from build123d import *

# Parameters (mm, degrees)
EXTRUDE003_DEPTH                     = 10
SKETCH009_R                          = 3.1
EXTRUDE002_DEPTH                     = 10
EXTRUDE001_DEPTH                     = 2.65
EXTRUDE001_ONTO_SKETCH005_ROLL_ANGLE = 90
EXTRUDE_DEPTH                        = 30
EXTRUDE_ONTO_SKETCH_ROLL_ANGLE       = 90
POCKET_DEPTH                         = 20.000966
SKETCH002_W                          = 9.15
SKETCH002_H                          = 3.1
POCKET001_DEPTH                      = 7
POCKET002_DEPTH                      = 3.739432
SKETCH004_R                          = 1.55
POCKET003_DEPTH                      = 7
SKETCH006_W                          = 6
SKETCH006_H                          = 4
POCKET004_DEPTH                      = 9.5
SKETCH007_R                          = 4.15
POCKET005_DEPTH                      = 14.611568
FILLET_R                             = 2.5
FILLET001_R                          = 1
FILLET002_R                          = 2
FILLET003_R                          = 1
CHAMFER_1_SIZE2                      = 16
CHAMFER_1_SIZE                       = 6
CHAMFER_2_SIZE2                      = 16
CHAMFER_2_SIZE                       = 6
CHAMFER001_SIZE                      = 5
SKETCH008_R                          = 1.55
POCKET006_DEPTH                      = 5.826
POCKET006_DEPTH_BACK                 = 6.476
FILLET004_R                          = 5


with BuildPart() as extrude003:
    # Sketch010 → Extrude003 (new body)
    with BuildSketch(Plane(origin=(0.325, 0, 0), x_dir=(0, -1, 0), z_dir=(-1, 0, 0))):
        Polygon((-21.103517, 11.668627), (-23.788196, 10.118627), (-23.788196, 7.018627), (-21.103517, 5.468627), (-18.418839, 7.018627), (-18.418839, 10.118627), align=None)
    extrude(amount=-EXTRUDE003_DEPTH)


with BuildPart() as extrude003_1:
    # Extrude003 placement: moved
    add(extrude003.part.moved(Location((2, 0, 0))))


with BuildPart() as extrude002:
    # Sketch009 → Extrude002 (new body)
    with BuildSketch(Plane.YZ.offset(-0.325)):
        with Locations((21.103517, 8.568627)):
            Circle(SKETCH009_R)
    extrude(amount=-EXTRUDE002_DEPTH)


with BuildPart() as extrude002_1:
    # Extrude002 placement: moved
    add(extrude002.part.moved(Location((-2, 0, 0))))


with BuildPart() as extrude001:
    # Sketch005 as drawn → Extrude001 (new)
    with BuildSketch(Plane.XY):
        Polygon((-2.75, -6.999966), (2.75, -6.999966), (2.75, -1.912252), (0, -0.324539), (-2.75, -1.912252), align=None)
    extrude(amount=-EXTRUDE001_DEPTH)


with BuildPart() as extrude001_1:
    # Extrude001 onto Sketch005 roll: moved
    add(extrude001.part.rotate(Axis((0, 0, 0), (1, 0, 0)), EXTRUDE001_ONTO_SKETCH005_ROLL_ANGLE))


with BuildPart() as extrude001_2:
    # Extrude001 onto Sketch005 placement: moved
    add(extrude001_1.part.moved(Location((0, 3.738432, 0))))


with BuildPart() as extrude001_3:
    # Extrude001 placement: moved
    add(extrude001_2.part.moved(Location((0, 3, 0))))


with BuildPart() as cut002:
    # Sketch as drawn → Extrude (new)
    with BuildSketch(Plane.XY):
        with BuildLine():
            ThreePointArc((-5.994013, 1.376339), (-6.110877, 0.692592), (-6.15, 3.4e-05))
            Line((-6.15, 3.4e-05), (-6.15, -6.999966))
            Line((-6.15, -6.999966), (6.15, -6.999966))
            Line((6.15, -6.999966), (6.15, 0))
            ThreePointArc((6.15, 0), (6.110879, 0.692575), (5.994013, 1.376339))
            Line((5.994013, 1.376339), (3.325, 13))
            Line((3.325, 13), (0.325, 13))
            Line((0.325, 13), (0.325, 0.945714))
            ThreePointArc((-0.325, 0.945714), (0, -1), (0.325, 0.945714))
            Line((-0.325, 13), (-0.325, 0.945714))
            Line((-3.325, 13), (-0.325, 13))
            Line((-5.994013, 1.376339), (-3.325, 13))
        make_face()
    extrude(amount=-EXTRUDE_DEPTH)


with BuildPart() as cut002_1:
    # Extrude onto Sketch roll: moved
    add(cut002.part.rotate(Axis((0, 0, 0), (1, 0, 0)), EXTRUDE_ONTO_SKETCH_ROLL_ANGLE))


with BuildPart() as cut002_2:
    # Extrude onto Sketch placement: moved
    add(cut002_1.part)

    # Sketch001 → Pocket (cut, through all)
    with BuildSketch(Plane(origin=(0, 0, -6.999966), x_dir=(1, 0, 0), z_dir=(0, 0, -1))):
        with BuildLine():
            Line((-6.15, 0), (6.15, 0))
            ThreePointArc((-6.15, 0), (0, -1.390023), (6.15, 0))
        make_face()
    extrude(amount=-POCKET_DEPTH, mode=Mode.SUBTRACT)

    # Sketch002 → Pocket001 (cut)
    with BuildSketch(Plane(origin=(0, 0, -6.999966), x_dir=(1, 0, 0), z_dir=(0, 0, -1))):
        with Locations((0, -2.188432)):
            Rectangle(SKETCH002_W, SKETCH002_H)
    extrude(amount=-POCKET001_DEPTH, mode=Mode.SUBTRACT)

    # Sketch003 → Pocket002 (cut, through all)
    with BuildSketch(Plane.XZ.offset(-3.738432)):
        Polygon((4.575, 3.4e-05), (-4.575, 3.4e-05), (0, 2.641412), align=None)
    extrude(amount=POCKET002_DEPTH, mode=Mode.SUBTRACT)

    # Sketch004 → Pocket003 (cut)
    with BuildSketch(Plane.XZ.offset(-3.738432)):
        with Locations((0, -3.499966)):
            Circle(SKETCH004_R)
    extrude(amount=-POCKET003_DEPTH, mode=Mode.SUBTRACT)

    # Cut: cut Extrude001
    add(extrude001_3.part, mode=Mode.SUBTRACT)

    # Sketch006 → Pocket004 (cut)
    with BuildSketch(Plane(origin=(0, 0, -6.999966), x_dir=(1, 0, 0), z_dir=(0, 0, -1))):
        with Locations((0, -13.388432)):
            Rectangle(SKETCH006_W, SKETCH006_H)
    extrude(amount=-POCKET004_DEPTH, mode=Mode.SUBTRACT)

    # Sketch007 → Pocket005 (cut)
    with BuildSketch(Plane(origin=(0, 30, 0), x_dir=(-1, 0, 0), z_dir=(0, 1, 0))):
        Circle(SKETCH007_R)
    extrude(amount=-POCKET005_DEPTH, mode=Mode.SUBTRACT)

    # Fillet
    fillet_edges = [cut002_2.edges().sort_by_distance(p)[0] for p in [
        (3, 13.388432, 2.500034),
        (-3, 13.388432, 2.500034),
    ]]
    fillet(fillet_edges, radius=FILLET_R)

    # Fillet001
    fillet001_edges = [cut002_2.edges().sort_by_distance(p)[0] for p in [
        (3, 11.388432, -3.499966),
        (2.267767, 11.388432, 1.767801),
        (0.4125, 11.388432, 2.500034),
        (-3, 11.388432, -3.499966),
        (-2.267767, 11.388432, 1.767801),
        (-0.4125, 11.388432, 2.500034),
    ]]
    fillet(fillet001_edges, radius=FILLET001_R)

    # Fillet002
    fillet002_edges = [cut002_2.edges().sort_by_distance(p)[0] for p in [
        (0, 15.388432, -4.15),
    ]]
    fillet(fillet002_edges, radius=FILLET002_R)

    # Fillet003
    fillet003_edges = [cut002_2.edges().sort_by_distance(p)[0] for p in [
        (3, 13.888432, -6.999966),
        (0, 15.388432, -6.999966),
        (2.707107, 11.681325, -6.999966),
        (0, 11.388432, -6.999966),
        (-3, 13.888432, -6.999966),
        (-2.707107, 11.681325, -6.999966),
    ]]
    fillet(fillet003_edges, radius=FILLET003_R)

    # Chamfer 1
    chamfer_1_edges = [cut002_2.edges().sort_by_distance(p)[0] for p in [
        (1.835295, 1.271761, 13),
    ]]
    chamfer_1_side = cut002_2.faces().sort_by_distance((3.310874, 1.001462, 3.000017))[0]
    chamfer(chamfer_1_edges, length=CHAMFER_1_SIZE, length2=CHAMFER_1_SIZE2, reference=chamfer_1_side)

    # Chamfer 2
    chamfer_2_edges = [cut002_2.edges().sort_by_distance(p)[0] for p in [
        (-1.835295, 1.271761, 13),
    ]]
    chamfer_2_side = cut002_2.faces().sort_by_distance((-3.310874, 1.001462, 3.000017))[0]
    chamfer(chamfer_2_edges, length=CHAMFER_2_SIZE, length2=CHAMFER_2_SIZE2, reference=chamfer_2_side)

    # Chamfer001
    chamfer001_edges = [cut002_2.edges().sort_by_distance(p)[0] for p in [
        (1.825, 30, 13),
        (-1.825, 30, 13),
    ]]
    chamfer(chamfer001_edges, length=CHAMFER001_SIZE)

    # Sketch008 → Pocket006 (cut, two sides)
    with BuildSketch(Plane.YZ.offset(-0.325)) as pocket006_sk:
        with Locations((21.103517, 8.568627)):
            Circle(SKETCH008_R)
    extrude(amount=-POCKET006_DEPTH, mode=Mode.SUBTRACT)
    extrude(pocket006_sk.sketch, amount=POCKET006_DEPTH_BACK, mode=Mode.SUBTRACT)

    # Fillet004
    fillet004_edges = [cut002_2.edges().sort_by_distance(p)[0] for p in [
        (1.825, 25, 13),
        (1.827249, 17.334877, 13),
        (2.399047, 30, 8),
        (-2.399047, 30, 8),
        (-1.825, 25, 13),
        (-1.827249, 17.334877, 13),
    ]]
    fillet(fillet004_edges, radius=FILLET004_R)

    # Cut001: cut Extrude002
    add(extrude002_1.part, mode=Mode.SUBTRACT)

    # Cut002: cut Extrude003
    add(extrude003_1.part, mode=Mode.SUBTRACT)


solid = cut002_2.part
Could you check a few things on this model? Use its own coordinates, in mm. A direction names the side the tool comes from. Round coordinates to 2 decimals unless told otherwise and drop trailing zeros. Order: outer loops, then holes, each group sorted by start corner. A loop starts at its lowest first (then second) coordinate and runs counter-clockwise, first axis right, second up.
Q1. Which directions (+Z, -Z, +X, -X, +Y, -Y) give clear straight access to the entire face, cutting with the end or side of a thin tool? Please do faces 5 (the face through (-2.75, 8, -4)), 6 (the face through (3.67, 22.46, 6.25)), 7 (the face through (2.42, 2.555, 1.244)), 8 (the face through (3, 15.388, 1)), 9 (the face through (2, 7.29, 9.25)).
Geometry says:
face 5: -Z
face 6: +X
face 7: -Z, -Y
face 8: +Y
face 9: +Z, -Y
Q2. Please list where these lines run through material, in increasing order: probe 1 along X at (y, z) = (7, 0); probe 2 along X at (y, z) = (13, -4.5); probe 3 along Y at (x, z) = (-2, -4.75).
Geometry says:
probe 1: x = -6.15 to -1, 1 to 6.15
probe 2: x = -6.15 to -3, 3 to 6.15
probe 3: y = 3.74 to 6.74, 9.39 to 11.39, 15.65 to 30
Q3. Imagine slicing it at A-A, the plane z = 11. List the corners of the cut face in (x, y) for me (3 decimals).
Geometry says:
outline: (-3.784, 11.768) arc R24.967 cw to (-0.325, 12.055) - (-0.325, 27) - (-3.784, 27) - (-3.784, 23.027) - (-2.325, 23.027) - (-2.325, 19.18) - (-3.784, 19.18) - close; (0.325, 12.055) arc R24.967 cw to (3.784, 11.768) - (3.784, 19.945) - (2.325, 19.945) - (2.325, 22.262) - (3.784, 22.262) - (3.784, 27) - (0.325, 27) - close
Q4. Thinking about a two-plate mould opening in Z: for faces 1 (the face through (2, 27, 11)), 2 (the face through (-3.393, 20.431, 5.542)), 3 (the face through (-1.848, 22.796, 3.716)), 4 (the face through (-1.71, 8.04, -1.31)), which applies, released by +Z, released by -Z, zero draft, split by the parting line, or undercut?
Geometry says:
face 1: released by +Z
face 2: undercut
face 3: undercut
face 4: released by -Z
Q5. I'm going to push flat-ended pins straight in: P1, Ø3, axis at x = 0.5, z = -2.5, coming from the +Y side; P2, Ø2, axis at x = -4, z = 0, coming from the -Y side; P3, Ø3.5, axis at y = 21.1, z = 8.57, coming from the -X side (3 decimals). Where does each tip first touch, or does it pass through?
Geometry says:
P1: stops at y = 11.39
P2: stops at y = 0.49
P3: stops at x = -2.325
Q6. Imagine slicing it at B-B, the plane y = 21.5. State how many separate pieces and enclosed holes the cut face has, then the cut area to 3 significant figures.
Geometry says:
separate pieces: 3
enclosed holes: 0
area: 115 mm2
